from build123d import *

# Parameters (mm, degrees)
ESQUISSE1_R                                = 50
BOSS_EXTRU_1_DEPTH                         = 5
ESQUISSE2_R                                = 26
ENL_V_MAT_EXTRU_1_DEPTH                    = 3
ESQUISSE3_R                                = 12.5
ENL_V_MAT_EXTRU_2_DEPTH                    = 71.887234394
CHAMBRAGE_POUR_VIS_T_TE_RONDE_BOMB_2_COUNT = 2
CHAMBRAGE_POUR_VIS_T_TE_RONDE_BOMB_2_PITCH = 49.497474683
CHAMBRAGE_POUR_VIS_T_TE_RONDE_BOMB_3_COUNT = 2
CHAMBRAGE_POUR_VIS_T_TE_RONDE_BOMB_3_PITCH = 70
CHAMBRAGE_POUR_VIS_T_TE_RONDE_BOMB_4_COUNT = 2
CHAMBRAGE_POUR_VIS_T_TE_RONDE_BOMB_4_PITCH = 49.497474683
D_GAGEMENT_M62_D                           = 6.6
BOSS_EXTRU_3_DEPTH                         = 5


with BuildPart() as part:
    # Esquisse1 → Boss.-Extru.1 (new body)
    with BuildSketch(Plane.XY):
        Circle(ESQUISSE1_R)
    extrude(amount=BOSS_EXTRU_1_DEPTH)

    # Esquisse2 → Enlèv. mat.-Extru.1 (cut)
    with BuildSketch(Plane.XY.offset(5)):
        Circle(ESQUISSE2_R)
    extrude(amount=-ENL_V_MAT_EXTRU_1_DEPTH, mode=Mode.SUBTRACT)

    # Esquisse3 → Enlèv. mat.-Extru.2 (cut, through all)
    with BuildSketch(Plane.XY.offset(5)):
        Circle(ESQUISSE3_R)
    extrude(amount=-ENL_V_MAT_EXTRU_2_DEPTH, mode=Mode.SUBTRACT)

    # Esquisse5 → Chambrage pour vis à tête ronde bombée M41 (revolve, cut)
    with BuildSketch(Plane(origin=(0, 35, 0), x_dir=(0, 1, 0), z_dir=(1, 0, 0))):
        Polygon((0, 0), (0, 5), (2.25, 5), (2.25, 3.125), (2.275, 3.1), (4.5, 3.1), (4.5, 0), align=None)
    chambrage_pour_vis_t_te_ronde_bomb_e_m = revolve(axis=Axis((0, 35, -6.35), (0, 0, 1)), mode=Mode.SUBTRACT)

    # Chambrage pour vis _ t_te ronde bomb 2: Chambrage pour vis à tête ronde bombée M41 ×2
    with Locations(*[Vector(-0.7071067811865476, -0.7071067811865476, 0) * (i * CHAMBRAGE_POUR_VIS_T_TE_RONDE_BOMB_2_PITCH) for i in range(1, CHAMBRAGE_POUR_VIS_T_TE_RONDE_BOMB_2_COUNT)]):
        add(chambrage_pour_vis_t_te_ronde_bomb_e_m, mode=Mode.SUBTRACT)

    # Chambrage pour vis _ t_te ronde bomb 3: Chambrage pour vis à tête ronde bombée M41 ×2
    with Locations(*[(0, -i * CHAMBRAGE_POUR_VIS_T_TE_RONDE_BOMB_3_PITCH, 0) for i in range(1, CHAMBRAGE_POUR_VIS_T_TE_RONDE_BOMB_3_COUNT)]):
        add(chambrage_pour_vis_t_te_ronde_bomb_e_m, mode=Mode.SUBTRACT)

    # Chambrage pour vis _ t_te ronde bomb 4: Chambrage pour vis à tête ronde bombée M41 ×2
    with Locations(*[Vector(0.7071067811865476, -0.7071067811865476, 0) * (i * CHAMBRAGE_POUR_VIS_T_TE_RONDE_BOMB_4_PITCH) for i in range(1, CHAMBRAGE_POUR_VIS_T_TE_RONDE_BOMB_4_COUNT)]):
        add(chambrage_pour_vis_t_te_ronde_bomb_e_m, mode=Mode.SUBTRACT)

    # Dégagement M62 (through all)
    with Locations(Plane.XY.offset(5)):
        with Locations((30.452660491, 27.824413184), (-27.824413184, 30.452660491), (-30.452660491, -27.824413184), (27.824413184, -30.452660491)):
            Hole(D_GAGEMENT_M62_D / 2)

    # Esquisse12 → Boss.-Extru.3 (add)
    with BuildSketch(Plane(origin=(0, 0, 0), x_dir=(-1, 0, 0), z_dir=(0, 0, -1))):
        with BuildLine():
            ThreePointArc((-61.551276684, 27.137434265), (-64.174792612, 24.35142904), (-64.059895327, 20.526319949))
            Line((-64.059895327, 20.526319949), (-45.598664842, -20.512478267))
            ThreePointArc((-45.598664842, -20.512478267), (-46.747637649, 17.738612524), (-20.512478495, 45.598664739))
            Line((-20.512478495, 45.598664739), (-61.551276684, 27.137434265))
        make_face()
        with BuildLine():
            ThreePointArc((20.51247781, -45.598665047), (-17.738612875, -46.747637515), (-45.598664842, -20.512478267))
            Line((-45.598664842, -20.512478267), (-27.137434265, -61.551276684))
            ThreePointArc((-27.137434265, -61.551276684), (-24.35142904, -64.174792612), (-20.526319949, -64.059895327))
            Line((-20.526319949, -64.059895327), (20.51247781, -45.598665047))
        make_face()
        with BuildLine():
            Line((20.526319949, 64.059895327), (-20.512478495, 45.598664739))
            ThreePointArc((-20.512478495, 45.598664739), (17.738612852, 46.747637524), (45.598665129, 20.512477628))
            Line((45.598665129, 20.512477628), (27.137434265, 61.551276684))
            ThreePointArc((27.137434265, 61.551276684), (24.35142904, 64.174792612), (20.526319949, 64.059895327))
        make_face()
        with BuildLine():
            ThreePointArc((45.598665129, 20.512477628), (46.747637391, -17.738613203), (20.51247781, -45.598665047))
            Line((20.51247781, -45.598665047), (61.551276684, -27.137434265))
            ThreePointArc((61.551276684, -27.137434265), (64.174792612, -24.35142904), (64.059895327, -20.526319949))
            Line((64.059895327, -20.526319949), (45.598665129, 20.512477628))
        make_face()
    extrude(amount=-BOSS_EXTRU_3_DEPTH)


solid = part.part
Design review of the part built by this model. Coordinates are the model's own, in mm. A direction names the side the tool comes from. Round coordinates to 2 decimals unless told otherwise and drop trailing zeros. Order: outer loops, then holes, each group sorted by start corner. A loop starts at its lowest first (then second) coordinate and runs counter-clockwise, first axis right, second up. Notation, with made-up numbers: M 29.5,37.5 L 61.5,37.5 A11 ccw 61.5,45.5 Z; hole C 14.5,45.25 d6. An arc over 180 degrees is marked long. Answer as CSV lines item,"result". Start each with the question number.
1) Add section C-C (y = 7.5). Give the boundary of the cut face in (x, z).
2) Add section D-D (y = -17.5). Give the boundary of the cut face in (x, z).
3) For pin 1 Ø3 at (x, z) = (43.5, 3) entering from +Y; pin 2 Ø1 at (y, z) = (-37, 1.5) entering from -X; pin 3 Ø5.5 at (x, y) = (-30.45, -27.82) entering from +Z; pin 4 Ø7 at (x, y) = (0, 35) entering from -Z, all flat-tipped, find the tip position at first contact; note any pin that passes through.
4) Tool access review of faces 5 (the face through (-20.633, -15.821, 3.521)), 6 (the face through (24.403, -64.155, 2.465)), 7 (the face through (-33, -2, 3.1)): name each direction out of +Z, -Z, +X, -X, +Y, -Y from which nothing blocks a thin tool from reaching the whole face with its end or side.
5) Wall thickness on line 1 along Y through (x, z) = (0, 4.1); line 2 along X through (y, z) = (28, 3.7); line 3 along X through (y, z) = (9, 2.6): over which ranges is each line inside the solid? List them lowest first. Write a range as [from, to].
6) Add section A-A (x = 0). Give the number of separate pieces and of enclosed holes in the cut face, then the cut area to 3 significant figures.
7) The part is to be moulded in two halves that separate along X. For faces 1 (the face through (0.86, -32.92, 4.05)), 2 (the face through (64.155, 24.403, 2.465)), 3 (the face through (-64.155, -24.403, 2.465)), 4 (the face through (-24.403, 64.155, 2.465)), say which applies: +X half, -X half, draft (parallel to the pull), parting line (faces both ways), or undercut.
Resolved:
1,outline,"M -51.45,0 L -10,0 L -10,2 L -24.89,2 L -24.89,5 L -51.45,5 Z; M 10,0 L 58.2,0 L 58.2,5 L 24.89,5 L 24.89,2 L 10,2 Z"
2,outline,"M -62.7,0 L 46.95,0 L 46.95,5 L 19.23,5 L 19.23,2 L -19.23,2 L -19.23,5 L -62.7,5 Z"
3,pin 1,"y = 35.93"
3,pin 2,"x = -40.74"
3,pin 3,"through"
3,pin 4,"z = 3.1"
4,face 5,"+Z"
4,face 6,"+Z, -Z, -Y"
4,face 7,"-Z"
5,line 1,"[-54.83, -37.25], [-32.75, -26], [26, 32.75], [37.25, 54.83]"
5,line 2,"[-42.23, -30.03], [-25.62, 27.16], [33.75, 59.63]"
5,line 3,"[-50.78, -24.39], [24.39, 58.87]"
6,separate pieces,"4"
6,enclosed holes,"0"
6,area,"269 mm^2"
7,face 1,"undercut"
7,face 2,"+X half"
7,face 3,"-X half"
7,face 4,"parting line"
